Read the model definition and answer for the solid it produces. Units are mm, in the model's axes. A direction names the side the tool comes from. Coordinates: 2 decimals unless noted, no trailing zeros. Write each loop counter-clockwise with the first axis right and the second up, starting at its lowest first coordinate (ties: lowest second). Pieces come first, ordered by that corner, then holes.
(1) Section D-D on y = 19.25 is taken. Write down the section's boundary in (x, z), then the cut area to 3 significant figures.
(2) Section C-C on z = -30 is taken. Write down the section's boundary in (x, y), then the cut area to 3 significant figures.
(3) Section B-B on y = 3.25 is taken. State how many separate pieces and enclosed holes the cut face has, then the cut area to 3 significant figures.
(4) Given pin 1 (4 mm diameter, centred on x = 44.5, z = -74, fed in from +Y); pin 2 (1 mm diameter, centred on y = 10.5, z = -14, fed in from -X); pin 3 (3 mm diameter, centred on x = 41, y = 3.5, fed in from +Z); pin 4 (3.5 mm diameter, centred on x = -46, z = 74.75, fed in from +Y), each flat-ended and moving along its own axis, determine where each tip first touches the part or whether it passes through.
(5) Section A-A on z = -74.75 is taken. Write down the section's boundary in (x, y) (3 decimals).
(6) The mould has two halves that part along X. Classify faces 1 (the cylindrical face through (-14.176, 7.818, -78.746)), 2 (the cylindrical face through (11.3, 7.8, 71.8)), 3 (the flat face through (15, 10, -77)), 4 (the cylindrical face through (24.51, 5.94, -67.65)): +X half, -X half, draft (parallel to the pull), parting line (faces both ways), or undercut.
(7) Which of the six approach directions +Z, -Z, +X, -X, +Y, -Y give full straight-line access (tool end or side, diameter ignored) to faces 5 (the flat face through (-42, 5, 70.5)), 6 (the flat face through (13, 12, 30)), 7 (the flat face through (21, 5, -89))?
(8) Find the intervals of material crossed by probe 1 along X at (y, z) = (18.5, -30); probe 2 along X at (y, z) = (1.5, -84.75); probe 3 along X at (y, z) = (13.25, 15), in increasing order.
from build123d import *

# Parameters (mm, degrees)
BOSS_EXTRUDE1_DEPTH                          = 10
FILLET1_R                                    = 10
SKETCH2_R                                    = 1.75
CUT_EXTRUDE1_DEPTH                           = 10
CBORE_FOR_M4_HEX_SOCKET_HEAD_CAP_SCR_2_COUNT = 2
CBORE_FOR_M4_HEX_SOCKET_HEAD_CAP_SCR_2_PITCH = 10
CBORE_FOR_M4_HEX_SOCKET_HEAD_CAP_SCR_3_COUNT = 2
CBORE_FOR_M4_HEX_SOCKET_HEAD_CAP_SCR_3_PITCH = 60
CBORE_FOR_M4_HEX_SOCKET_HEAD_CAP_SCR_4_COUNT = 2
CBORE_FOR_M4_HEX_SOCKET_HEAD_CAP_SCR_4_PITCH = 152.099474029
CBORE_FOR_M4_HEX_SOCKET_HEAD_CAP_SCR_5_COUNT = 2
CBORE_FOR_M4_HEX_SOCKET_HEAD_CAP_SCR_5_PITCH = 161.939031737
CBORE_FOR_M4_HEX_SOCKET_HEAD_CAP_SCR_6_COUNT = 2
CBORE_FOR_M4_HEX_SOCKET_HEAD_CAP_SCR_6_PITCH = 162.67836365
CBORE_FOR_M4_HEX_SOCKET_HEAD_CAP_SCR_7_COUNT = 2
CBORE_FOR_M4_HEX_SOCKET_HEAD_CAP_SCR_7_PITCH = 152.886395732
CBORE_FOR_M4_HEX_SOCKET_HEAD_CAP_SCR_8_COUNT = 2
CBORE_FOR_M4_HEX_SOCKET_HEAD_CAP_SCR_8_PITCH = 60.827625303
FILLET2_R                                    = 2.5
FILLET3_R                                    = 2.5
SKETCH5_W                                    = 43
SKETCH5_H                                    = 121
BOSS_EXTRUDE2_DEPTH                          = 12
CHAMFER1_SIZE                                = 5
SKETCH7_R                                    = 2.25
CUT_EXTRUDE2_DEPTH                           = 10
SKETCH8_R                                    = 2.25
CUT_EXTRUDE3_DEPTH                           = 10


with BuildPart() as part:
    # Sketch1 → Boss-Extrude1 (new body)
    with BuildSketch(Plane(origin=(0, 0, 0), x_dir=(1, 0, 0), z_dir=(0, 1, 0))):
        Polygon((-21.5, -89), (21.5, -89), (21.5, 70.5), (53.5, 70.5), (53.5, 89), (-21.5, 89), (-21.5, -70.5), (-53.5, -70.5), (-53.5, -89), align=None)
    extrude(amount=BOSS_EXTRUDE1_DEPTH)

    # Fillet1
    fillet1_edges = [part.edges().sort_by_distance(p)[0] for p in [
        (-21.5, 5, 70.5),
        (-21.5, 5, -89),
        (21.5, 5, -70.5),
        (21.5, 5, 89),
    ]]
    fillet(fillet1_edges, radius=FILLET1_R)

    # Sketch2 → Cut-Extrude1 (cut)
    with BuildSketch(Plane(origin=(0, 10, 0), x_dir=(1, 0, 0), z_dir=(0, 1, 0))):
        with Locations(Location((-14, 74.75, 0), (0, 0, 270))):
            Circle(SKETCH2_R)
        with Locations(Location((-14, 84.75, 0), (0, 0, 270))):
            Circle(SKETCH2_R)
        with Locations(Location((46, 74.75, 0), (0, 0, 270))):
            Circle(SKETCH2_R)
        with Locations(Location((46, 84.75, 0), (0, 0, 270))):
            Circle(SKETCH2_R)
        with Locations(Location((-46, -74.75, 0), (0, 0, 270))):
            Circle(SKETCH2_R)
        with Locations(Location((-46, -84.75, 0), (0, 0, 270))):
            Circle(SKETCH2_R)
        with Locations(Location((14, -74.75, 0), (0, 0, 270))):
            Circle(SKETCH2_R)
        with Locations(Location((14, -84.75, 0), (0, 0, 270))):
            Circle(SKETCH2_R)
    extrude(amount=-CUT_EXTRUDE1_DEPTH, mode=Mode.SUBTRACT)

    # Sketch4 → CBORE for M4 Hex Socket Head Cap Screw1 (revolve, cut)
    with BuildSketch(Plane(origin=(-14, 10, -74.75), x_dir=(0, 0, 1), z_dir=(1, 0, 0))):
        Polygon((0, 0), (0, 11.351936393), (2.25, 10), (2.25, 4.4), (4, 4.4), (4, 0.025), (4.025, 0), align=None)
    cbore_for_m4_hex_socket_head_cap_screw1 = revolve(axis=Axis((-14, 16.35, -74.75), (0, -1, 0)), mode=Mode.SUBTRACT)

    # CBORE for M4 Hex Socket Head Cap Scr 2: CBORE for M4 Hex Socket Head Cap Screw1 ×2
    with Locations(*[(0, 0, -i * CBORE_FOR_M4_HEX_SOCKET_HEAD_CAP_SCR_2_PITCH) for i in range(1, CBORE_FOR_M4_HEX_SOCKET_HEAD_CAP_SCR_2_COUNT)]):
        add(cbore_for_m4_hex_socket_head_cap_screw1, mode=Mode.SUBTRACT)

    # CBORE for M4 Hex Socket Head Cap Scr 3: CBORE for M4 Hex Socket Head Cap Screw1 ×2
    with Locations(*[(i * CBORE_FOR_M4_HEX_SOCKET_HEAD_CAP_SCR_3_PITCH, 0, 0) for i in range(1, CBORE_FOR_M4_HEX_SOCKET_HEAD_CAP_SCR_3_COUNT)]):
        add(cbore_for_m4_hex_socket_head_cap_screw1, mode=Mode.SUBTRACT)

    # CBORE for M4 Hex Socket Head Cap Scr 4: CBORE for M4 Hex Socket Head Cap Screw1 ×2
    with Locations(*[Vector(0.1840900514527529, 0, 0.9829093818639248) * (i * CBORE_FOR_M4_HEX_SOCKET_HEAD_CAP_SCR_4_PITCH) for i in range(1, CBORE_FOR_M4_HEX_SOCKET_HEAD_CAP_SCR_4_COUNT)]):
        add(cbore_for_m4_hex_socket_head_cap_screw1, mode=Mode.SUBTRACT)

    # CBORE for M4 Hex Socket Head Cap Scr 5: CBORE for M4 Hex Socket Head Cap Screw1 ×2
    with Locations(*[Vector(0.1729045783441913, 0, 0.9849385802107751) * (i * CBORE_FOR_M4_HEX_SOCKET_HEAD_CAP_SCR_5_PITCH) for i in range(1, CBORE_FOR_M4_HEX_SOCKET_HEAD_CAP_SCR_5_COUNT)]):
        add(cbore_for_m4_hex_socket_head_cap_screw1, mode=Mode.SUBTRACT)

    # CBORE for M4 Hex Socket Head Cap Scr 6: CBORE for M4 Hex Socket Head Cap Screw1 ×2
    with Locations(*[Vector(-0.19670716671795496, 0, 0.9804622841097942) * (i * CBORE_FOR_M4_HEX_SOCKET_HEAD_CAP_SCR_6_PITCH) for i in range(1, CBORE_FOR_M4_HEX_SOCKET_HEAD_CAP_SCR_6_COUNT)]):
        add(cbore_for_m4_hex_socket_head_cap_screw1, mode=Mode.SUBTRACT)

    # CBORE for M4 Hex Socket Head Cap Scr 7: CBORE for M4 Hex Socket Head Cap Screw1 ×2
    with Locations(*[Vector(-0.20930573872668637, 0, 0.9778502481137263) * (i * CBORE_FOR_M4_HEX_SOCKET_HEAD_CAP_SCR_7_PITCH) for i in range(1, CBORE_FOR_M4_HEX_SOCKET_HEAD_CAP_SCR_7_COUNT)]):
        add(cbore_for_m4_hex_socket_head_cap_screw1, mode=Mode.SUBTRACT)

    # CBORE for M4 Hex Socket Head Cap Scr 8: CBORE for M4 Hex Socket Head Cap Screw1 ×2
    with Locations(*[Vector(0.9863939238321426, 0, -0.1643989873053641) * (i * CBORE_FOR_M4_HEX_SOCKET_HEAD_CAP_SCR_8_PITCH) for i in range(1, CBORE_FOR_M4_HEX_SOCKET_HEAD_CAP_SCR_8_COUNT)]):
        add(cbore_for_m4_hex_socket_head_cap_screw1, mode=Mode.SUBTRACT)

    # Fillet2
    # the kernel refuses this fillet: 2.5 mm, written as the material it takes off along each edge
    with BuildSketch(Plane(origin=(-13.754801439, 5.6, -88.742477635), x_dir=(0.9990847033117879, 0, -0.042775642699985884), z_dir=(0, 1, 0))) as fillet2_piece_1:
        with BuildLine():
            CenterArc((5.91336471, -2.497711758), FILLET2_R, 87.548388178, 105.618498276)
            Line((3.479087926, -3.067182162), (3.235660248, -3.124129202))
            ThreePointArc((3.235660248, -3.124129202), (2.064143441, -1.165399671), (-0.025984683, -0.248645925))
            Line((-0.025984683, -0.248645925), (-0.045899922, 0.245750274))
            ThreePointArc((-0.045899922, 0.245750274), (2.274447223, 0.410607251), (6.030997727, 0.249771176))
            Line((6.030997727, 0.249771176), (6.020303816, 0))
        make_face()
    extrude(amount=19.425759541, mode=Mode.SUBTRACT)
    with BuildSketch(Plane(origin=(-17.087010961, 5.6, -87.293690886), x_dir=(-0.5524220177087732, 0, 0.8335645831911094), z_dir=(0, 1, 0))) as fillet2_piece_2:
        with BuildLine():
            CenterArc((6.697143458, 2.309687979), FILLET2_R, 165.124054411, 127.376595494)
            ThreePointArc((4.280933593, 2.951505625), (2.685480046, 0.685252699), (0, 0))
            ThreePointArc((0, 0), (3.826939119, -0.761248083), (7.653878238, 0))
        make_face()
    extrude(amount=23.509695594, mode=Mode.SUBTRACT)

    # Fillet3
    # the kernel refuses this fillet: 2.5 mm, written as the material it takes off along each edge
    with BuildSketch(Plane(origin=(13.75480144, 5.6, 88.742477635), x_dir=(-0.7777172566996915, 0, -0.6286142446934416), z_dir=(0, 1, 0))) as fillet3_piece_1:
        with BuildLine():
            CenterArc((6.087462048, 2.036971289), FILLET3_R, 128.947957862, 105.618498276)
            Line((4.515926436, 3.98126443), (4.358772875, 4.175693744))
            ThreePointArc((4.358772875, 4.175693744), (1.434562202, 1.812109205), (-0.196946455, 0.153987317))
            Line((-0.196946455, 0.153987317), (0.144939573, -0.203697129))
            ThreePointArc((0.144939573, -0.203697129), (2.319033161, 0.490845938), (4.49312675, -0.203697129))
            Line((4.49312675, -0.203697129), (4.638066322, 0))
        make_face()
    extrude(amount=19.425759541, mode=Mode.SUBTRACT)
    with BuildSketch(Plane(origin=(17.087010961, 5.6, 87.293690886), x_dir=(-0.018344711955799436, 0, -0.9998317216128216), z_dir=(0, 1, 0))) as fillet3_piece_2:
        with BuildLine():
            CenterArc((6.824719559, -1.89989263), FILLET3_R, 130.539588182, 127.376595494)
            ThreePointArc((6.30136363, -4.344498645), (2.718581752, -2.798977477), (0, 0))
            ThreePointArc((0, 0), (2.599893165, -0.960171793), (5.19978633, 0))
        make_face()
    extrude(amount=23.509695594, mode=Mode.SUBTRACT)

    # Sketch5 → Boss-Extrude2 (add)
    with BuildSketch(Plane(origin=(0, 10, 0), x_dir=(1, 0, 0), z_dir=(0, 1, 0))):
        Rectangle(SKETCH5_W, SKETCH5_H)
    extrude(amount=BOSS_EXTRUDE2_DEPTH)

    # Chamfer1
    # the kernel refuses this chamfer: 5 mm, written as the material it adds along each edge
    with BuildSketch(Plane(origin=(34.35841494, 10, -60.5), x_dir=(0, -0.027495876610586317, -0.9996219169112968), z_dir=(-1, 0, 0))) as chamfer1_piece_1_section:
        Polygon((CHAMFER1_SIZE * 0.999621916911, -CHAMFER1_SIZE * 0.0274958766106), (-CHAMFER1_SIZE * 0.0274958766106, -CHAMFER1_SIZE * 0.999621916911), (0, 0), align=None)
    chamfer1_piece_1 = extrude(amount=55.85841494, mode=Mode.PRIVATE)
    chamfer1_piece_1 = chamfer1_piece_1 - Plane(origin=(31.5, 10.859011568, -60.5), x_dir=(0, 0, -1), z_dir=(0, 1, 0)) * Cylinder(10, 132, mode=Mode.PRIVATE)
    add(chamfer1_piece_1)
    with BuildSketch(Plane(origin=(-34.35841494, 10, 60.5), x_dir=(0, -0.027495876610586317, 0.9996219169112968), z_dir=(1, 0, 0))) as chamfer1_piece_2_section:
        Polygon((CHAMFER1_SIZE * 0.999621916911, -CHAMFER1_SIZE * 0.0274958766106), (-CHAMFER1_SIZE * 0.0274958766106, -CHAMFER1_SIZE * 0.999621916911), (0, 0), align=None)
    chamfer1_piece_2 = extrude(amount=55.85841494, mode=Mode.PRIVATE)
    chamfer1_piece_2 = chamfer1_piece_2 - Plane(origin=(-31.5, 10.859011568, 60.5), x_dir=(0, 0, 1), z_dir=(0, 1, 0)) * Cylinder(10, 132, mode=Mode.PRIVATE)
    add(chamfer1_piece_2)

    # Sketch7 → Cut-Extrude2 (cut)
    with BuildSketch(Plane(origin=(0, 22, 0), x_dir=(1, 0, 0), z_dir=(0, 1, 0))):
        with Locations(Location((0, 0, 0), (0, 0, 270))):
            Circle(SKETCH7_R)
    extrude(amount=-CUT_EXTRUDE2_DEPTH, mode=Mode.SUBTRACT)

    # Sketch8 → Cut-Extrude3 (cut)
    with BuildSketch(Plane(origin=(0, 22, 0), x_dir=(1, 0, 0), z_dir=(0, 1, 0))):
        with Locations(Location((12.5, 30, 0), (0, 0, 270))):
            Circle(SKETCH8_R)
        with Locations(Location((-12.5, 30, 0), (0, 0, 270))):
            Circle(SKETCH8_R)
        with Locations(Location((-12.5, -30, 0), (0, 0, 270))):
            Circle(SKETCH8_R)
        with Locations(Location((12.5, -30, 0), (0, 0, 270))):
            Circle(SKETCH8_R)
    extrude(amount=-CUT_EXTRUDE3_DEPTH, mode=Mode.SUBTRACT)


solid = part.part
Response:
1. outline: (-21.5, -60.5) - (21.5, -60.5) - (21.5, 60.5) - (-21.5, 60.5) - close; hole circle Ø4.5 at (-12.5, -30); hole circle Ø4.5 at (-12.5, 30); hole circle Ø4.5 at (0, 0); hole circle Ø4.5 at (12.5, -30); hole circle Ø4.5 at (12.5, 30)
1. area: 5,120 mm2
2. outline: (-21.5, 0) - (21.5, 0) - (21.5, 22) - (14.75, 22) - (14.75, 12) - (10.25, 12) - (10.25, 22) - (-10.25, 22) - (-10.25, 12) - (-14.75, 12) - (-14.75, 22) - (-21.5, 22) - close
2. area: 856 mm2
3. separate pieces: 1
3. enclosed holes: 8
3. area: 8,710 mm2
4. pin 1: stops at y = 5.6
4. pin 2: stops at x = -21.5
4. pin 3: stops at z = -70.5
4. pin 4: passes through
5. outline: (-21.5, 0) - (-16.25, 0) - (-16.25, 5.6) - (-18, 5.6) - (-18, 9.975) - (-18.025, 10) - (-21.5, 10) - close; (-11.75, 0) - (43.75, 0) - (43.75, 5.6) - (42, 5.6) - (42, 9.975) - (41.975, 10) - (-9.975, 10) - (-10, 9.975) - (-10, 5.6) - (-11.75, 5.6) - close; (48.25, 0) - (53.5, 0) - (53.5, 10) - (50.025, 10) - (50, 9.975) - (50, 5.6) - (48.25, 5.6) - close
6. face 1: undercut
6. face 2: undercut
6. face 3: draft
6. face 4: +X half
7. face 5: -Z, -X, +Y, -Y
7. face 6: +Y
7. face 7: -Z, +X, -X, +Y, -Y
8. probe 1: x = -21.5 to -14.75, -10.25 to 10.25, 14.75 to 21.5
8. probe 2: x = -19.68 to -16.25, -11.75 to 43.75, 48.25 to 53.5
8. probe 3: x = -21.5 to 21.5
